The listing builds one solid part. Answer for the finished solid, in the listing's coordinates (mm). Face numbers are marked on the shaded views. A direction names the side the tool comes from. Coordinates: 2 decimals unless noted, no trailing zeros. Write each loop counter-clockwise with the first axis right and the second up, starting at its lowest first coordinate (ties: lowest second). Pieces come first, ordered by that corner, then holes. Notation, with made-up numbers: M 88,17.5 L 130,17.5 A37 cw 130,55.5 Z; hole C 74,-20 d3. An arc over 180 degrees is marked long. Put each result on its own line as item: value. Start each with the question number.
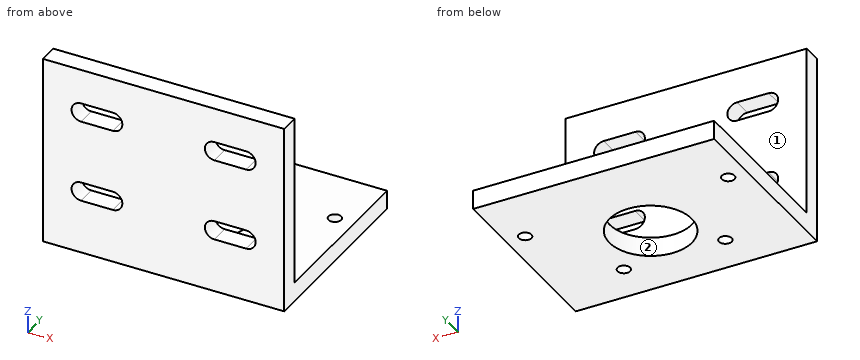
```python
from build123d import *

# Parameters (mm, degrees)
SKETCH2_W           = 38
SKETCH2_H           = 30
BOSS_EXTRUDE1_DEPTH = 3
SKETCH3_W           = 38
SKETCH3_H           = 3
BOSS_EXTRUDE2_DEPTH = 27
SKETCH4_R           = 6.5
CUT_EXTRUDE1_DEPTH  = 27
CUT_EXTRUDE2_DEPTH  = 37.262928729
SKETCH6_R           = 1
CUT_EXTRUDE3_DEPTH  = 45.609416046


with BuildPart() as part:
    # Sketch2 → Boss-Extrude1 (new body)
    with BuildSketch(Plane(origin=(0, 0, 0), x_dir=(1, 0, 0), z_dir=(0, 1, 0))):
        Rectangle(SKETCH2_W, SKETCH2_H)
    extrude(amount=BOSS_EXTRUDE1_DEPTH)

    # Sketch3 → Boss-Extrude2 (add)
    with BuildSketch(Plane(origin=(0, 3, 0), x_dir=(1, 0, 0), z_dir=(0, 1, 0))):
        with Locations((0, 13.5)):
            Rectangle(SKETCH3_W, SKETCH3_H)
    extrude(amount=BOSS_EXTRUDE2_DEPTH)

    # Sketch4 → Cut-Extrude1 (cut)
    with BuildSketch(Plane.XY.offset(-12)):
        with Locations((0, 13.35)):
            Circle(SKETCH4_R)
    extrude(amount=-CUT_EXTRUDE1_DEPTH, mode=Mode.SUBTRACT)

    # Sketch5 → Cut-Extrude2 (cut, through all)
    with BuildSketch(Plane(origin=(0, 3, 0), x_dir=(1, 0, 0), z_dir=(0, 1, 0))):
        with BuildLine():
            Line((-13, 6.5), (-8, 6.5))
            ThreePointArc((-8, 6.5), (-6.5, 5), (-8, 3.5))
            Line((-8, 3.5), (-13, 3.5))
            ThreePointArc((-13, 3.5), (-14.5, 5), (-13, 6.5))
        make_face()
        with BuildLine():
            Line((8, 6.5), (13, 6.5))
            ThreePointArc((13, 6.5), (14.5, 5), (13, 3.5))
            Line((13, 3.5), (8, 3.5))
            ThreePointArc((8, 3.5), (6.5, 5), (8, 6.5))
        make_face()
        with BuildLine():
            Line((8, -6.5), (13, -6.5))
            ThreePointArc((13, -6.5), (14.5, -8), (13, -9.5))
            Line((13, -9.5), (8, -9.5))
            ThreePointArc((8, -9.5), (6.5, -8), (8, -6.5))
        make_face()
        with BuildLine():
            Line((-13, -6.5), (-8, -6.5))
            ThreePointArc((-8, -6.5), (-6.5, -8), (-8, -9.5))
            Line((-8, -9.5), (-13, -9.5))
            ThreePointArc((-13, -9.5), (-14.5, -8), (-13, -6.5))
        make_face()
    extrude(amount=-CUT_EXTRUDE2_DEPTH, mode=Mode.SUBTRACT)

    # Sketch6 → Cut-Extrude3 (cut, through all)
    with BuildSketch(Plane.XY.offset(-12)):
        with Locations((16, 20.35)):
            Circle(SKETCH6_R)
        with Locations((-16, 20.35)):
            Circle(SKETCH6_R)
        with Locations((-8, 6.35)):
            Circle(SKETCH6_R)
        with Locations((8, 6.35)):
            Circle(SKETCH6_R)
    extrude(amount=-CUT_EXTRUDE3_DEPTH, mode=Mode.SUBTRACT)


solid = part.part
```
1) For the marked faces 1 and 2, determine the directions among +Z, -Z, +X, -X, +Y, -Y from which every point of the face is accessible in a straight line to the end or side of a thin tool.
2) Given pin 1 Ø2.5 at (x, y) = (-8, 6.35) entering from +Z; pin 2 Ø5 at (x, z) = (-11, -3.5) entering from +Y, each flat-ended and moving along its own axis, determine where each tip first touches the part or whether it passes through.
3) A cutting plane is placed at A-A on z = 8. Write down the section's boundary in (x, y).
4) Straight lines are drawn through the part: probe 1 along Y at (x, z) = (-8, -13.05); probe 2 along Y at (x, z) = (0, -13.25); probe 3 along Z at (x, y) = (-13.5, 25.25). For each, find the intervals that lie inside material, in ascending order.
5) A cutting plane is placed at B-B on y = 20.35. Write down the section's boundary in (x, z).
6) A cutting plane is placed at D-D on x = 6. Write down the section's boundary in (y, z).
7) A cutting plane is placed at C-C on x = 10. Write down the section's boundary in (y, z), then the cut area to 3 significant figures.
Answers follow:
1. face 1: +Z, +X, -X, +Y
1. face 2: +Z, -Z
2. pin 1: stops at z = -12
2. pin 2: stops at y = 3
3. outline: M -19,0 L -14.5,0 L -14.5,3 L -19,3 Z; M -6.5,0 L 6.5,0 L 6.5,3 L -6.5,3 Z; M 14.5,0 L 19,0 L 19,3 L 14.5,3 Z
4. probe 1: y = 0 to 5.35, 7.35 to 30
4. probe 2: y = 0 to 6.85, 19.85 to 30
4. probe 3: z = -15 to -12
5. outline: M -19,-15 L -17,-15 L -17,-12 L -19,-12 Z; M -15,-15 L 15,-15 L 15,-12 L -15,-12 Z; M 17,-15 L 19,-15 L 19,-12 L 17,-12 Z
6. outline: M 0,-15 L 10.85,-15 L 10.85,-12 L 3,-12 L 3,15 L 0,15 Z; M 15.85,-15 L 30,-15 L 30,-12 L 15.85,-12 Z
7. outline: M 0,-15 L 30,-15 L 30,-12 L 3,-12 L 3,-6.5 L 0,-6.5 Z; M 0,-3.5 L 3,-3.5 L 3,6.5 L 0,6.5 Z; M 0,9.5 L 3,9.5 L 3,15 L 0,15 Z
7. area: 153 mm²
